```python
from build123d import *

# Parameters (mm, degrees)
SKETCH_1_W          = 27
SKETCH_1_H          = 10.8
EXTRUDE_1_DEPTH     = 12
SKETCH_2_W          = 3.9
SKETCH_2_H          = 3.9
CUT_EXTRUDE_1_DEPTH = 10.5
FILLET_1_R          = 2
SKETCH_3_R          = 1.1
CUT_EXTRUDE_2_DEPTH = 40.5
SKETCH_4_W          = 27
SKETCH_4_H          = 10.8
SKETCH_4_W_2        = 19.2
SKETCH_4_H_2        = 8
CUT_EXTRUDE_3_DEPTH = 4


with BuildPart() as part:
    # 스케치1 → 보스-돌출1 (new body)
    with BuildSketch(Plane(origin=(0, 0, 0), x_dir=(1, 0, 0), z_dir=(0, 1, 0))):
        Rectangle(SKETCH_1_W, SKETCH_1_H)
    extrude(amount=EXTRUDE_1_DEPTH)

    # 스케치2 → 컷-돌출1 (cut)
    with BuildSketch(Plane(origin=(0, 12, 0), x_dir=(1, 0, 0), z_dir=(0, 1, 0))):
        with Locations((-11.55, 3.45)):
            Rectangle(SKETCH_2_W, SKETCH_2_H)
        with Locations((11.55, -3.45)):
            Rectangle(SKETCH_2_W, SKETCH_2_H)
    extrude(amount=-CUT_EXTRUDE_1_DEPTH, mode=Mode.SUBTRACT)

    # 필렛1
    fillet_1_edges = [part.edges().sort_by_distance(p)[0] for p in [
        (-9.6, 6.75, -1.5),
        (9.6, 6.75, 1.5),
    ]]
    fillet(fillet_1_edges, radius=FILLET_1_R)

    # 스케치3 → 컷-돌출2 (cut)
    with BuildSketch(Plane(origin=(0, 12, 0), x_dir=(1, 0, 0), z_dir=(0, 1, 0))):
        with Locations((-11.7, 3.3)):
            Circle(SKETCH_3_R)
        with Locations((11.7, -3.3)):
            Circle(SKETCH_3_R)
    extrude(amount=-CUT_EXTRUDE_2_DEPTH, mode=Mode.SUBTRACT)

    # 스케치4 → 컷-돌출3 (cut)
    with BuildSketch(Plane(origin=(0, 12, 0), x_dir=(1, 0, 0), z_dir=(0, 1, 0))):
        Rectangle(SKETCH_4_W, SKETCH_4_H)
        Rectangle(SKETCH_4_W_2, SKETCH_4_H_2, mode=Mode.SUBTRACT)
    extrude(amount=-CUT_EXTRUDE_3_DEPTH, mode=Mode.SUBTRACT)


solid = part.part
```
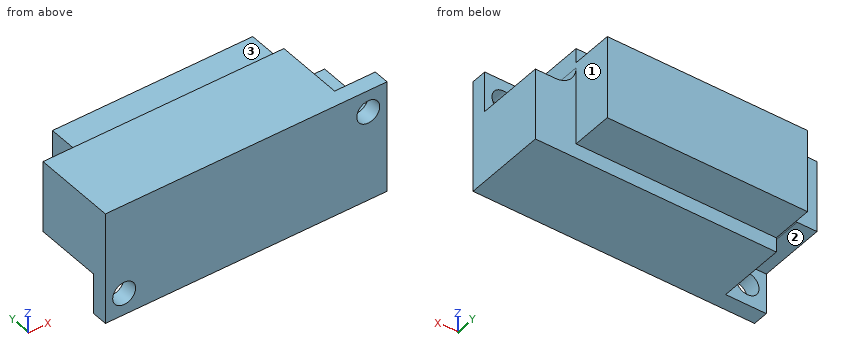
Model file for the job. Use its own axes, mm. Face numbers are marked on the shaded views. A direction names the side the tool comes from. Coordinates: 2 decimals unless noted, no trailing zeros. Order: outer loops, then holes, each group sorted by start corner. A loop starts at its lowest first (then second) coordinate and runs counter-clockwise, first axis right, second up. Notation, with made-up numbers: (7, 58.5) - (17, 58.5) arc R27 ccw to (17, 90.5) - close; hole circle Ø11 at (-38.5, -26.5). An arc over 180 degrees is marked (long way). Return JSON: item names as keys, results as strings. Group by question number.
1) Probe line 1 (X direction, y = 0.45, z = 3.3); line 2 (X direction, y = 0.45, z = -3.3); line 3 (Z direction, x = -11.7, y = 0.8). List the from-to ranges inside material, lowest first. Write a range as from..to.
2) Saw through at A-A, the plane y = 4.5. Write the cut outline in (x, z).
3) Saw through at B-B, the plane x = 9. Write the cut outline in (y, z).
4) Saw through at D-D, the plane z = -2.75. Write the cut outline in (x, y), plus the area to 3 significant figures.
5) Tool access for the marked faces 1, 2 and 3: list every direction of +Z, -Z, +X, -X, +Y, -Y with a clear straight run to the whole face (end or side of a thin tool).
6) Saw through at C-C, the plane z = 1. Write the cut outline in (x, y), plus the area to 3 significant figures.
7) Flat gauge pins, fed straight in: P1, Ø1, axis at x = 2, y = 9, coming from the +Z side; P2, Ø1.2, axis at x = -12, z = -3, coming from the +Y side; P3, Ø2, axis at x = 12.5, y = 4, coming from the +Z side; P4, Ø1.5, axis at x = -12.5, y = 3.5, coming from the -Z side. Where does each tip first touch, or does it go through?
Values found:
{
 "1": {"line 1": "x = -13.5..10.6, 12.8..13.5", "line 2": "x = -13.5..-12.8, -10.6..13.5", "line 3": "z = -5.4..-4.4, -2.2..5.4"},
 "2": {"outline": "(-13.5, -1.5) - (-11.6, -1.5) arc R2 cw to (-9.6, -3.5) - (-9.6, -5.4) - (13.5, -5.4) - (13.5, 1.5) - (11.6, 1.5) arc R2 cw to (9.6, 3.5) - (9.6, 5.4) - (-13.5, 5.4) - close"},
 "3": {"outline": "(0, -5.4) - (8, -5.4) - (8, -4) - (12, -4) - (12, 4) - (8, 4) - (8, 5.4) - (0, 5.4) - close"},
 "4": {"outline": "(-13.5, 0) - (-12.65, 0) - (-12.65, 1.5) - (-13.5, 1.5) - close; (-10.75, 0) - (13.5, 0) - (13.5, 8) - (9.6, 8) - (9.6, 12) - (-9.6, 12) - (-9.6, 8) - (-9.75, 8) - (-9.75, 1.5) - (-10.75, 1.5) - close", "area": "266 mm²"},
 "5": {"face 1": "+Z, +X, +Y", "face 2": "-Z, -X, +Y", "face 3": "+Z, +X, -X, +Y"},
 "6": {"outline": "(-13.5, 0) - (13.5, 0) - (13.5, 8) - (9.6, 8) - (9.6, 12) - (-9.6, 12) - (-9.6, 8) - (-13.5, 8) - close", "area": "293 mm²"},
 "7": {"P1": "stops at z = 4", "P2": "passes through", "P3": "stops at z = 1.5", "P4": "stops at z = -1.5"}
}
